Design review of the part built by this model. Coordinates are the model's own, in mm. A direction names the side the tool comes from. Round coordinates to 2 decimals unless told otherwise and drop trailing zeros. Write each loop counter-clockwise with the first axis right and the second up, starting at its lowest first coordinate (ties: lowest second). Pieces come first, ordered by that corner, then holes. Notation, with made-up numbers: (78, -38.5) - (118, -38.5) arc R6 ccw to (118, -30.5) - close; hole circle Ø3 at (36.5, 38). An arc over 180 degrees is marked (long way). Use one line per item in the form item = value.
```python
from build123d import *

# Parameters (mm, degrees)
BOSS_EXTRUDE2_DEPTH = 57.15
SKETCH8_R           = 6.35
CUT_EXTRUDE8_DEPTH  = 91.948
SKETCH6_R           = 6.35
CUT_EXTRUDE9_DEPTH  = 91.948


with BuildPart() as part:
    # Sketch1 → Boss-Extrude2 (new body)
    with BuildSketch(Plane.XY):
        with BuildLine():
            Line((-152.4, 2.2186447), (0, 0))
            Line((0, 0), (0, 12.7))
            Line((0, 12.7), (-31.75, 12.7))
            Line((-31.75, 12.7), (-31.75, 44.45))
            Line((-31.75, 44.45), (-43.829743935, 44.75146974))
            ThreePointArc((-43.829743935, 44.75146974), (-43.825200034, 44.441370306), (-43.823685352, 44.131241281))
            ThreePointArc((-43.823685352, 44.131241281), (-76.675806516, 12.400375725), (-107.247170639, 46.334155203))
            Line((-107.247170639, 46.334155203), (-120.65, 46.6686447))
            Line((-120.65, 46.6686447), (-120.65, 14.9186447))
            Line((-120.65, 14.9186447), (-152.4, 14.9186447))
            Line((-152.4, 14.9186447), (-152.4, 2.2186447))
        make_face()
    extrude(amount=BOSS_EXTRUDE2_DEPTH)

    # Sketch8 → Cut-Extrude8 (cut)
    with BuildSketch(Plane(origin=(0, 14.9186447, 0), x_dir=(1, 0, 0), z_dir=(0, 1, 0))):
        with Locations(Location((-135.898685352, -28.575, 0), (0, 0, 270))):
            Circle(SKETCH8_R)
    extrude(amount=-CUT_EXTRUDE8_DEPTH, mode=Mode.SUBTRACT)

    # Sketch6 → Cut-Extrude9 (cut)
    with BuildSketch(Plane(origin=(0, 12.7, 0), x_dir=(1, 0, 0), z_dir=(0, 1, 0))):
        with Locations(Location((-15.248685352, -28.575, 0), (0, 0, 270))):
            Circle(SKETCH6_R)
    extrude(amount=-CUT_EXTRUDE9_DEPTH, mode=Mode.SUBTRACT)


solid = part.part
```
Q1. To check wall thickness, follow line 1 along X through (y, z) = (9, 34); line 2 along X through (y, z) = (34.5, 23); line 3 along X through (y, z) = (37, 7). State the ranges of each line that lie inside material, in increasing order. Write a range as from..to.
Calculated:
line_1 = -152.4..-139.2, -132.6..-18.55, -11.95..0
line_2 = -120.65..-105.83, -45.32..-31.75
line_3 = -120.65..-106.51, -44.63..-31.75
Q2. Machinability: for faces 4 (the flat face through (-16, 12.7, 22)), 5 (the flat face through (-120.65, 31, 28)), 6 (the cylindrical face through (-14.97, 6.49, 22.23)), which of the approach directions +Z, -Z, +X, -X, +Y, -Y give a long, thin tool a straight path to every point of the face, cutting with its end or side? Answer none if there is none.
Calculated:
face_4 = +Z, -Z, +X, +Y
face_5 = +Z, -Z, -X, +Y
face_6 = +Y, -Y
Q3. We need section B-B on y = 33. Write out the cut boundary in (x, z).
Calculated:
outline = (-120.65, 0) - (-105.31, 0) - (-105.31, 57.15) - (-120.65, 57.15) - close; (-45.84, 0) - (-31.75, 0) - (-31.75, 57.15) - (-45.84, 57.15) - close
Q4. We need section C-C on z = 32. Write out the cut boundary in (x, y), then the cut area to 3 significant figures.
Calculated:
outline = (-152.4, 2.22) - (-141.25, 2.06) - (-141.25, 14.92) - (-152.4, 14.92) - close; (-130.55, 1.9) - (-20.6, 0.3) - (-20.6, 12.7) - (-31.75, 12.7) - (-31.75, 44.45) - (-43.83, 44.75) arc R31.75 cw to (-43.82, 44.13) arc R31.75 cw (long way) to (-107.25, 46.33) - (-120.65, 46.67) - (-120.65, 14.92) - (-130.55, 14.92) - close; (-9.9, 0.14) - (0, 0) - (0, 12.7) - (-9.9, 12.7) - close
area = 2,810 mm2
Q5. We need section A-A on x = -133. Write out the cut boundary in (y, z).
Calculated:
outline = (1.94, 0) - (14.92, 0) - (14.92, 22.93) - (1.94, 22.93) - close; (1.94, 34.22) - (14.92, 34.22) - (14.92, 57.15) - (1.94, 57.15) - close
Q6. We need section D-D on z = 25. Write out the cut boundary in (x, y).
Calculated:
outline = (-152.4, 2.22) - (-141.15, 2.05) - (-141.15, 14.92) - (-152.4, 14.92) - close; (-130.65, 1.9) - (-20.5, 0.3) - (-20.5, 12.7) - (-31.75, 12.7) - (-31.75, 44.45) - (-43.83, 44.75) arc R31.75 cw to (-43.82, 44.13) arc R31.75 cw (long way) to (-107.25, 46.33) - (-120.65, 46.67) - (-120.65, 14.92) - (-130.65, 14.92) - close; (-10, 0.15) - (0, 0) - (0, 12.7) - (-10, 12.7) - close
Q7. Draft analysis for pull direction Z (two halves, no side actions). For faces 1 (the flat face through (-31.75, 28, 28)), 2 (the flat face through (-77, 8, 0)), 3 (the cylindrical face through (-131.6, 8.5, 23.9)), state which applies: released by +Z, released by -Z, zero draft, split by the parting line, or undercut.
Calculated:
face_1 = zero draft
face_2 = released by -Z
face_3 = undercut
Q8. For P1, Ø2, axis at x = -79.5, z = 12, coming from the +Y side; P2, Ø9.5, axis at x = -138.5, z = 14.5, coming from the +Y side; P3, Ø6, axis at y = 18.5, z = 12.5, coming from the +X side; P4, Ø3, axis at x = -96, y = 13.5, coming from the -Z side, all flat-tipped, find the tip position at first contact; note any pin that passes through.
Calculated:
P1 = 12.77
P2 = 14.92
P3 = -31.75
P4 = 0
